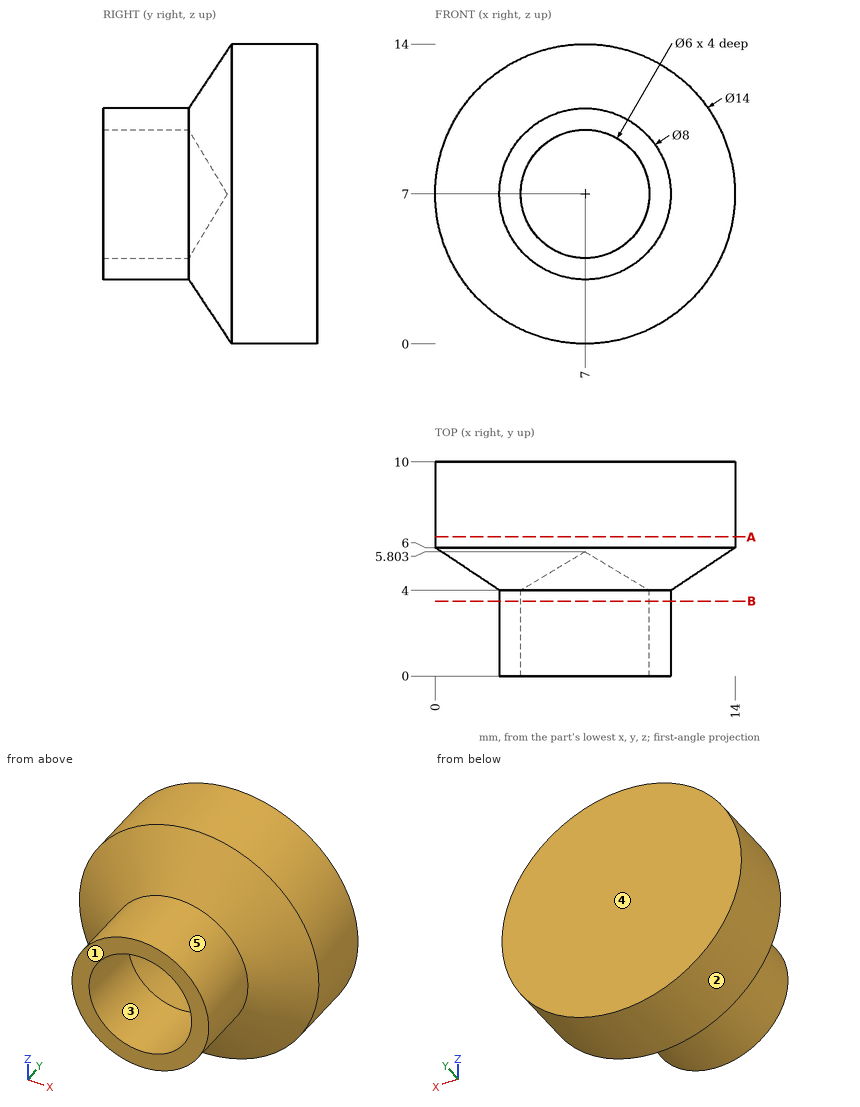
Source: three-view drawing plus pictorial views. Frame: mm from the lowest corner of the part. A direction names the side the tool comes from. Give positions to 0.01 mm unless a question says otherwise; leave off trailing zeros. Order: outer loops, then holes, each group sorted by start corner. A loop starts at its lowest first (then second) coordinate and runs counter-clockwise, first axis right, second up. Notation, with made-up numbers: (12, -33) - (65, -33) arc R21 ccw to (65, 2) - close; hole circle Ø8 at (15.5, 20.25). An arc over 180 degrees is marked (long way). Put each result on its own line as item: value.
Item 1: Section query A-A, the plane y = 6.5. Return loops of the section in (x, z), then the cut area to 3 significant figures.
Found:
outline: circle Ø14 at (7, 7)
area: 154 mm^2
Item 2: Draft query along Z for the marked faces 1, 2 and 3. Return one class per face: +Z half, -Z half, draft (parallel to the pull), parting line (faces both ways), or undercut.
Found:
face 1: draft
face 2: parting line
face 3: undercut
Item 3: Contact query for flat-ended pins moving along their axis: pin 1 (4 mm diameter, centred on y = 3.5, z = 3.5, fed in from -X); pin 2 (4 mm diameter, centred on x = 4, y = 6, fed in from +Z); pin 3 (1 mm diameter, centred on x = 6, y = 3.5, fed in from -Z). Output: stop coordinate, or through.
Found:
pin 1: stops at x = 1.62
pin 2: stops at z = 13.93
pin 3: stops at z = 3.03
Item 4: Ray query, L1, parallel to X at y = 2.1, z = 7; L2, parallel to Z at x = 9.25, y = 3.75 (1 decimal); L3, parallel to X at y = 1.5, z = 5.5. Return the intervals inside material, ascending. Write a range as from..to.
Found:
L1: x = 3..4, 10..11
L2: z = 3.7..5, 9..10.3
L3: x = 3.29..4.4, 9.6..10.71
Item 5: Section query B-B, the plane y = 3.5. Return loops of the section in (x, z).
Found:
outline: circle Ø8 at (7, 7); hole circle Ø6 at (7, 7)
Item 6: Access query for the marked faces 4 and 5. Directions: +Z, -Z, +X, -X, +Y, -Y. A direction counts if a zero-diameter tool reaches every point of the face in a straight line with its end or side. Return the directions, or none.
Found:
face 4: +Z, -Z, +X, -X, +Y
face 5: -Y
